from build123d import *

# Parameters (mm, degrees)
F0_R     = 63.5
F0_R_2   = 12.7
F1_DEPTH = 6.35
F2_T     = 5.08
F3_SIZE  = 2.54
F4_R     = 12.7
F4_R_2   = 8.001
F5_DEPTH = 6.35


# Not quite as in the source:
# - a shell that OpenCascade refuses in one call is made with other operations: the cavity is built on its own and cut out


with BuildPart() as f1:
    # F0 (on Top) → F1 (new body)
    with BuildSketch(Plane.XY):
        Circle(F0_R)
        with BuildLine():
            ThreePointArc((4.4125195695, -52.5690356897), (0, -56.9815552592), (-4.4125195695, -52.5690356897))
            Line((-4.4125195695, -52.5690356897), (-4.4125195695, -23.4904065728))
            ThreePointArc((-4.4125195695, -23.4904065728), (0, -19.0778870033), (4.4125195695, -23.4904065728))
            Line((4.4125195695, -23.4904065728), (4.4125195695, -52.5690356897))
        make_face(mode=Mode.SUBTRACT)
        with BuildLine():
            ThreePointArc((-48.6325804131, -20.4412808959), (-54.1926794379, -17.608268941), (-51.359667483, -12.0481699162))
            Line((-51.359667483, -12.0481699162), (-23.7042477765, -3.0623793459))
            ThreePointArc((-23.7042477765, -3.0623793459), (-18.1441487516, -5.8953913008), (-20.9771607065, -11.4554903256))
            Line((-20.9771607065, -11.4554903256), (-48.6325804131, -20.4412808959))
        make_face(mode=Mode.SUBTRACT)
        with BuildLine():
            ThreePointArc((-27.3295005859, -45.1228571793), (-33.4929178341, -46.0990465706), (-34.4691072254, -39.9356293225))
            Line((-34.4691072254, -39.9356293225), (-17.3771178736, -16.4105241938))
            ThreePointArc((-17.3771178736, -16.4105241938), (-11.2137006254, -15.4343348024), (-10.2375112341, -21.5977520506))
            Line((-10.2375112341, -21.5977520506), (-27.3295005859, -45.1228571793))
        make_face(mode=Mode.SUBTRACT)
        with BuildLine():
            ThreePointArc((34.4691072254, -39.9356293225), (33.4929178341, -46.0990465706), (27.3295005859, -45.1228571793))
            Line((27.3295005859, -45.1228571793), (10.2375112341, -21.5977520506))
            ThreePointArc((10.2375112341, -21.5977520506), (11.2137006254, -15.4343348024), (17.3771178736, -16.4105241938))
            Line((17.3771178736, -16.4105241938), (34.4691072254, -39.9356293225))
        make_face(mode=Mode.SUBTRACT)
        with BuildLine():
            ThreePointArc((51.359667483, -12.0481699162), (54.1926794379, -17.608268941), (48.6325804131, -20.4412808959))
            Line((48.6325804131, -20.4412808959), (20.9771607065, -11.4554903256))
            ThreePointArc((20.9771607065, -11.4554903256), (18.1441487516, -5.8953913008), (23.7042477765, -3.0623793459))
            Line((23.7042477765, -3.0623793459), (51.359667483, -12.0481699162))
        make_face(mode=Mode.SUBTRACT)
        with BuildLine():
            ThreePointArc((-51.359667483, 12.0481699162), (-54.1926794379, 17.608268941), (-48.6325804131, 20.4412808959))
            Line((-48.6325804131, 20.4412808959), (-20.9771607065, 11.4554903256))
            ThreePointArc((-20.9771607065, 11.4554903256), (-18.1441487516, 5.8953913008), (-23.7042477765, 3.0623793459))
            Line((-23.7042477765, 3.0623793459), (-51.359667483, 12.0481699162))
        make_face(mode=Mode.SUBTRACT)
        with BuildLine():
            ThreePointArc((-34.4691072254, 39.9356293225), (-33.4929178341, 46.0990465706), (-27.3295005859, 45.1228571793))
            Line((-27.3295005859, 45.1228571793), (-10.2375112341, 21.5977520506))
            ThreePointArc((-10.2375112341, 21.5977520506), (-11.2137006254, 15.4343348024), (-17.3771178736, 16.4105241938))
            Line((-17.3771178736, 16.4105241938), (-34.4691072254, 39.9356293225))
        make_face(mode=Mode.SUBTRACT)
        Circle(F0_R_2, mode=Mode.SUBTRACT)
        with BuildLine():
            ThreePointArc((27.3295005859, 45.1228571793), (33.4929178341, 46.0990465706), (34.4691072254, 39.9356293225))
            Line((34.4691072254, 39.9356293225), (17.3771178736, 16.4105241938))
            ThreePointArc((17.3771178736, 16.4105241938), (11.2137006254, 15.4343348024), (10.2375112341, 21.5977520506))
            Line((10.2375112341, 21.5977520506), (27.3295005859, 45.1228571793))
        make_face(mode=Mode.SUBTRACT)
        with BuildLine():
            ThreePointArc((48.6325804131, 20.4412808959), (54.1926794379, 17.608268941), (51.359667483, 12.0481699162))
            Line((51.359667483, 12.0481699162), (23.7042477765, 3.0623793459))
            ThreePointArc((23.7042477765, 3.0623793459), (18.1441487516, 5.8953913008), (20.9771607065, 11.4554903256))
            Line((20.9771607065, 11.4554903256), (48.6325804131, 20.4412808959))
        make_face(mode=Mode.SUBTRACT)
        with BuildLine():
            Line((4.4125195695, 52.5690356897), (4.4125195695, 23.4904065728))
            ThreePointArc((4.4125195695, 23.4904065728), (0, 19.0778870033), (-4.4125195695, 23.4904065728))
            Line((-4.4125195695, 23.4904065728), (-4.4125195695, 52.5690356897))
            ThreePointArc((-4.4125195695, 52.5690356897), (0, 56.9815552592), (4.4125195695, 52.5690356897))
        make_face(mode=Mode.SUBTRACT)
    extrude(amount=F1_DEPTH)

    # F2: shell of thickness 5.08, made by hand


with BuildPart() as f2_core1:
    # F2_t2: copy of F1
    add(f1.part)

    # the walls: a layer under each face that stays
    f2_faces = [f2_core1.faces().sort_by_distance(p)[0] for p in [
        (-63.5, 0, 3.175),
        (4.4125195695, -38.0297211313, 3.175),
        (0, -56.9815552592, 3.175),
        (-4.4125195695, -38.0297211313, 3.175),
        (0, -19.0778870033, 3.175),
        (-18.1441487516, -5.8953913008, 3.175),
        (-34.8048705598, -15.9483856108, 3.175),
        (-54.1926794379, -17.608268941, 3.175),
        (-37.5319576298, -7.555274631, 3.175),
        (-18.78350591, -33.3603046149, 3.175),
        (-33.4929178341, -46.0990465706, 3.175),
        (-25.9231125495, -28.1730767581, 3.175),
        (-11.2137006254, -15.4343348024, 3.175),
        (11.2137006254, -15.4343348024, 3.175),
        (25.9231125495, -28.1730767581, 3.175),
        (33.4929178341, -46.0990465706, 3.175),
        (18.78350591, -33.3603046149, 3.175),
        (18.1441487516, -5.8953913008, 3.175),
        (37.5319576298, -7.555274631, 3.175),
        (54.1926794379, -17.608268941, 3.175),
        (34.8048705598, -15.9483856108, 3.175),
        (-37.5319576298, 7.555274631, 3.175),
        (-54.1926794379, 17.608268941, 3.175),
        (-34.8048705598, 15.9483856108, 3.175),
        (-18.1441487516, 5.8953913008, 3.175),
        (-25.9231125495, 28.1730767581, 3.175),
        (-33.4929178341, 46.0990465706, 3.175),
        (-18.78350591, 33.3603046149, 3.175),
        (-11.2137006254, 15.4343348024, 3.175),
        (-12.7, 0, 3.175),
        (11.2137006254, 15.4343348024, 3.175),
        (18.78350591, 33.3603046149, 3.175),
        (33.4929178341, 46.0990465706, 3.175),
        (25.9231125495, 28.1730767581, 3.175),
        (18.1441487516, 5.8953913008, 3.175),
        (34.8048705598, 15.9483856108, 3.175),
        (54.1926794379, 17.608268941, 3.175),
        (37.5319576298, 7.555274631, 3.175),
        (0, 19.0778870033, 3.175),
        (-4.4125195695, 38.0297211313, 3.175),
        (0, 56.9815552592, 3.175),
        (4.4125195695, 38.0297211313, 3.175),
        (-42.3333333333, -42.3333333333, 6.35),
    ]]
    thicken(f2_faces, amount=-F2_T, mode=Mode.SUBTRACT)


with BuildPart() as f1_1:
    add(f1.part)

    # what is left inside the walls is the cavity
    f2_cavity = [f2_core1.part.solids().sort_by_distance(p)[0] for p in [
        (17.763773, -48.3307, 1.2192),
        (38.738777, -34.159737, 1.2192),
        (44.569219, -3.470458, 1.2192),
        (38.738777, 26.107791, 1.2192),
        (12.812871, 48.3307, 1.2192),
        (-22.714676, 48.3307, 0.0508),
        (-38.738777, 26.107791, 0.0508),
        (-44.569219, -3.470458, 0.0508),
        (-38.738777, -34.159737, 1.2192),
        (-17.763773, -48.3307, 0.0508),
    ]]
    add(f2_cavity, mode=Mode.SUBTRACT)

    # F3
    f3_edges = [f1_1.edges().sort_by_distance(p)[0] for p in [
        (-63.5, 0, 6.35),
    ]]
    chamfer(f3_edges, length=F3_SIZE)

    # F4 (on face) → F5 (join)
    with BuildSketch(Plane.XY.offset(6.35)):
        Circle(F4_R)
        Circle(F4_R_2, mode=Mode.SUBTRACT)
    extrude(amount=-F5_DEPTH)


solid = f1_1.part
Check sheet for the modelled part. Datum: model origin and axes. Units: mm. A direction names the side the tool comes from. Round coordinates to 2 decimals unless told otherwise and drop trailing zeros. Order: outer loops, then holes, each group sorted by start corner. A loop starts at its lowest first (then second) coordinate and runs counter-clockwise, first axis right, second up.
Q1. Set-up check for faces 1 (the face through (-48, 0, 1.27)), 2 (the face through (-37.338, 7.492, 3.131)): record each of +Z, -Z, +X, -X, +Y, -Y from which the full face is reachable in a straight line by a thin tool's end or side.
Filled sheet:
face 1: -Z
face 2: +Z, -Z
Q2. Cross-section at B-B, the plane z = 2.5. Give the number of separate pieces and of enclosed holes in the cut face, plus the area to 3 significant figures.
Filled sheet:
separate pieces: 1
enclosed holes: 11
area: 9,290 mm2
Q3. Scan lines: L1, parallel to Y at x = 0, z = 2; L2, parallel to Y at x = -23.5, z = 5.5; L3, parallel to X at y = 24, z = 4.5. Record each from-to range of solid material in increasing order.
Filled sheet:
L1: y = -63.5 to -56.98, -19.08 to -8, 8 to 19.08, 56.98 to 63.5
L2: y = -57.17 to -39.85, -24.84 to -12.28, -3 to 3, 12.28 to 24.84, 39.85 to 57.17
L3: x = -58.04 to -22.89, -11.98 to -4.41, 4.41 to 11.98, 22.89 to 58.04
Q4. Draft check along Y on faces 3 (the face through (-13.77, -61.99, 1.88)), 4 (the face through (-36.113, 21.715, 0.626)), 5 (the face through (37.338, -7.492, 3.131)). Enter one of: pulls with the +Y half, pulls with the -Y half, needs draft (parallel to the pull), parting line crosses it, or undercut.
Filled sheet:
face 3: parting line crosses it
face 4: undercut
face 5: undercut
Q5. Depth check by flat-ended pin: P1, Ø1, axis at y = -45, z = 0.5, coming from the +X side; P2, Ø3, axis at y = -19.5, z = 1.5, coming from the +X side; P3, Ø0.6, axis at y = 46, z = 1, coming from the -X side. Enter the tip coordinate at first touch or a pass-through.
Filled sheet:
P1: stops at x = 45.3
P2: stops at x = 60.9
P3: stops at x = -44.09
Q6. Cross-section at A-A, the plane x = 0. Enter the section's corners in (y, z), plus the area to 3 significant figures.
Filled sheet:
outline: (-63.5, 0) - (-56.98, 0) - (-56.98, 6.35) - (-60.96, 6.35) - (-63.5, 3.81) - close; (-19.08, 0) - (-8, 0) - (-8, 6.35) - (-19.08, 6.35) - close; (8, 0) - (19.08, 0) - (19.08, 6.35) - (8, 6.35) - close; (56.98, 0) - (63.5, 0) - (63.5, 3.81) - (60.96, 6.35) - (56.98, 6.35) - close
area: 217 mm2
